from build123d import *

# Parameters (mm, degrees)
SKETCH1_W           = 350
SKETCH1_H           = 300
BOSS_EXTRUDE1_DEPTH = 30
SKETCH3_W           = 40
SKETCH3_H           = 260
CUT_EXTRUDE1_DEPTH  = 31
FILLET1_R           = 10


with BuildPart() as part:
    # Sketch1 → Boss-Extrude1 (new body)
    with BuildSketch(Plane(origin=(0, 0, 0), x_dir=(1, 0, 0), z_dir=(0, 1, 0))):
        with Locations((175, -150)):
            Rectangle(SKETCH1_W, SKETCH1_H)
    extrude(amount=BOSS_EXTRUDE1_DEPTH)

    # Sketch3 → Cut-Extrude1 (cut, through all)
    with BuildSketch(Plane(origin=(0, 0, 0), x_dir=(-1, 0, 0), z_dir=(0, -1, 0))):
        with Locations((-40, -150)):
            Rectangle(SKETCH3_W, SKETCH3_H)
        with Locations((-107.5, -150.391320706)):
            Rectangle(SKETCH3_W, SKETCH3_H)
        with Locations((-175, -150.782641412)):
            Rectangle(SKETCH3_W, SKETCH3_H)
        with Locations((-242.5, -151.173962118)):
            Rectangle(SKETCH3_W, SKETCH3_H)
        with Locations((-310, -151.565282825)):
            Rectangle(SKETCH3_W, SKETCH3_H)
    extrude(amount=-CUT_EXTRUDE1_DEPTH, mode=Mode.SUBTRACT)

    # Fillet1
    fillet1_edges = [part.edges().sort_by_distance(p)[0] for p in [
        (0, 15, 300),
        (0, 15, 0),
        (350, 15, 0),
        (350, 15, 300),
    ]]
    fillet(fillet1_edges, radius=FILLET1_R)


solid = part.part
Input: part model. Units: mm. Frame: model coordinates. A direction names the side the tool comes from. Give positions to 0.01 mm unless a question says otherwise; leave off trailing zeros. Order: outer loops, then holes, each group sorted by start corner. A loop starts at its lowest first (then second) coordinate and runs counter-clockwise, first axis right, second up.
Q1. Ray query, probe 1 along X at (y, z) = (8.25, 99); probe 2 along Z at (x, y) = (48.5, 7.75); probe 3 along Z at (x, y) = (309, 9.5). Return the intervals inside material, ascending.
Checked values:
probe 1: x = 0 to 20, 60 to 87.5, 127.5 to 155, 195 to 222.5, 262.5 to 290, 330 to 350
probe 2: z = 0 to 20, 280 to 300
probe 3: z = 0 to 21.57, 281.57 to 300
Q2. Section A-A on y = 14. Output: boundary loops of the cut face in (x, z).
Checked values:
outline: (0, 10) arc R10 ccw to (10, 0) - (340, 0) arc R10 ccw to (350, 10) - (350, 290) arc R10 ccw to (340, 300) - (10, 300) arc R10 ccw to (0, 290) - close; hole (20, 20) - (60, 20) - (60, 280) - (20, 280) - close; hole (87.5, 20.39) - (127.5, 20.39) - (127.5, 280.39) - (87.5, 280.39) - close; hole (155, 20.78) - (195, 20.78) - (195, 280.78) - (155, 280.78) - close; hole (222.5, 21.17) - (262.5, 21.17) - (262.5, 281.17) - (222.5, 281.17) - close; hole (290, 21.57) - (330, 21.57) - (330, 281.57) - (290, 281.57) - close
Q3. Draft query along X for faces 3 (the flat face through (350, 15, 152)), 4 (the flat face through (175, 15, 20.783)), 5 (the flat face through (173, 15, 0)). Return one class per face: +X half, -X half, draft (parallel to the pull), parting line (faces both ways), or undercut.
Checked values:
face 3: +X half
face 4: undercut
face 5: draft
Q4. Section B-B on z = 111. Output: boundary loops of the cut face in (x, y).
Checked values:
outline: (0, 0) - (20, 0) - (20, 30) - (0, 30) - close; (60, 0) - (87.5, 0) - (87.5, 30) - (60, 30) - close; (127.5, 0) - (155, 0) - (155, 30) - (127.5, 30) - close; (195, 0) - (222.5, 0) - (222.5, 30) - (195, 30) - close; (262.5, 0) - (290, 0) - (290, 30) - (262.5, 30) - close; (330, 0) - (350, 0) - (350, 30) - (330, 30) - close
Q5. Set-up query: faces 1 (the cylindrical face through (346.99, 15.21, 2.85)), 2 (the flat face through (310, 15, 281.565)). Return all of +Z, -Z, +X, -X, +Y, -Y with unobstructed straight access to the full face (end or side cutting, diameter ignored); none if empty.
Checked values:
face 1: -Z, +X, +Y, -Y
face 2: +Y, -Y
Q6. Section C-C on x = 162. Output: boundary loops of the cut face in (y, z).
Checked values:
outline: (0, 0) - (30, 0) - (30, 20.78) - (0, 20.78) - close; (0, 280.78) - (30, 280.78) - (30, 300) - (0, 300) - close
